Check sheet for the drawn part. Datum: minimum x, y, z corner. Units: mm. A direction names the side the tool comes from. Coordinates: 2 decimals unless noted, no trailing zeros. Write each loop counter-clockwise with the first axis right and the second up, starting at its lowest first coordinate (ties: lowest second). Pieces come first, ordered by that corner, then holes. Notation, with made-up numbers: (31.5, 20.25) - (53.5, 20.25) arc R3 cw to (53.5, 25.25) - close; hole circle Ø7 at (75, -36.5). An arc over 180 degrees is marked (long way). Use one line per item in the form item = value. Start each with the question number.
1. Cross-section at A-A on z = 69. Record the boundary of the cut face in (x, y).
2. Go/stop test with flat-tipped pins: pin 1 Ø2 at (x, z) = (2.5, 48.5) entering from +Y; pin 2 Ø2 at (x, z) = (5.5, 67.5) entering from +Y; pin 3 Ø3.5 at (y, z) = (4.5, 68.5) entering from +X; pin 4 Ø3 at (y, z) = (8.5, 33) entering from -X. Record where each tip stops, or that it passes through.
3. Cross-section at C-C on z = 26.5. Record the boundary of the cut face in (x, y), then the cut area to 3 significant figures.
4. Draft check along Z on the marked faces 1, 2, 3 and 4. Enter one of: +Z half, -Z half, draft (parallel to the pull), parting line (faces both ways), or undercut.
5. Cross-section at B-B on x = 5.8. Record the boundary of the cut face in (y, z).
6. Tool access check on the marked faces 5, 6 and 7. Record the directions out of +Z, -Z, +X, -X, +Y, -Y that give a thin tool (end or side, any length) a straight path to the whole face; none if there is none.
7. Scan lines: line 1 along Z through (x, y) = (1.5, 9.25); line 2 along Z through (x, y) = (8.5, 7.75); line 3 along Y through (x, z) = (6.25, 69). Record each from-to range of solid material in increasing order.
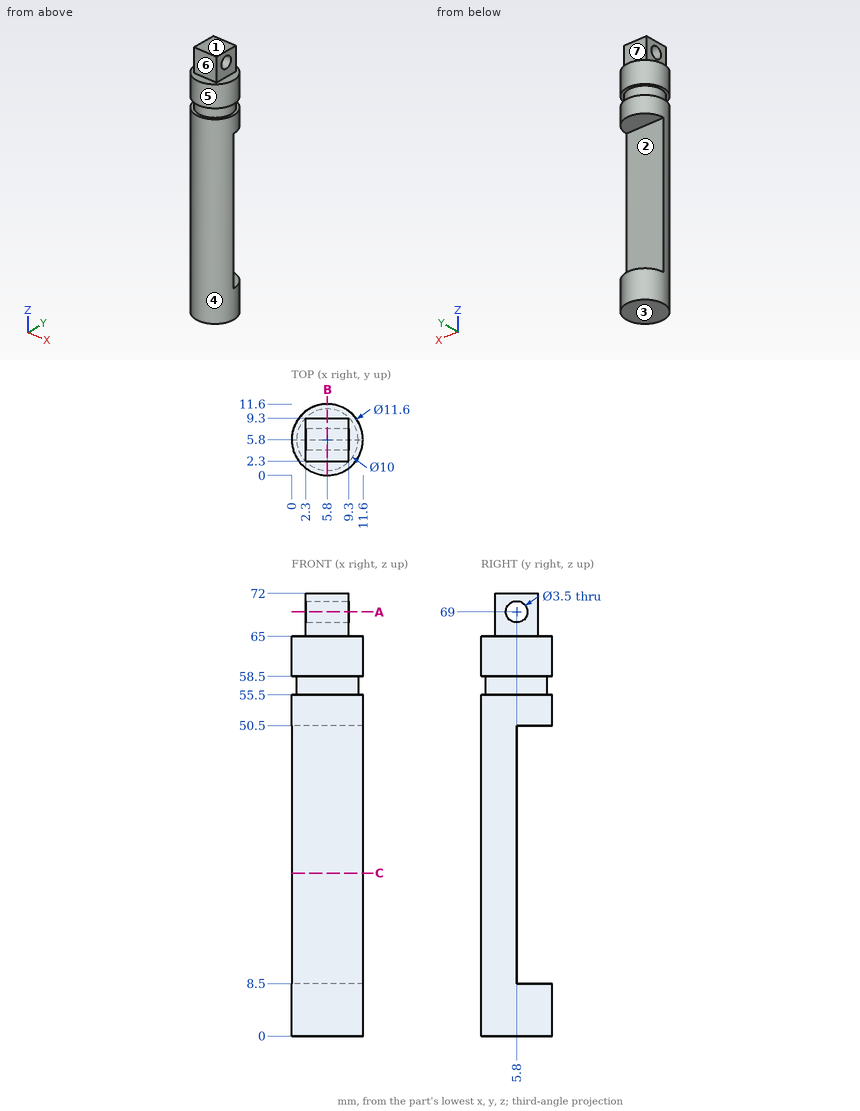
Final values:
q1.outline = (2.3, 2.3) - (9.3, 2.3) - (9.3, 4.05) - (2.3, 4.05) - close; (2.3, 7.55) - (9.3, 7.55) - (9.3, 9.3) - (2.3, 9.3) - close
q2.pin_1 = 5.8
q2.pin_2 = 9.3
q2.pin_3 = 9.3
q2.pin_4 = through
q3.outline = (0, 5.8) arc R5.8 ccw to (11.6, 5.8) - close
q3.area = 52.8 mm²
q4.face_1 = +Z half
q4.face_2 = undercut
q4.face_3 = -Z half
q4.face_4 = draft
q5.outline = (0, 0) - (11.6, 0) - (11.6, 8.5) - (5.8, 8.5) - (5.8, 50.5) - (11.6, 50.5) - (11.6, 55.5) - (10.8, 55.5) - (10.8, 58.5) - (11.6, 58.5) - (11.6, 65) - (9.3, 65) - (9.3, 72) - (2.3, 72) - (2.3, 65) - (0, 65) - (0, 58.5) - (0.8, 58.5) - (0.8, 55.5) - (0, 55.5) - close; hole circle Ø3.5 at (5.8, 69)
q6.face_5 = +Z, -Z
q6.face_6 = +Z, +X, -X, -Y
q6.face_7 = +Z, +X, -X, +Y
q7.line_1 = 0 to 8.5, 50.5 to 55.5, 58.5 to 65
q7.line_2 = 0 to 8.5, 50.5 to 72
q7.line_3 = 2.3 to 4.05, 7.55 to 9.3
